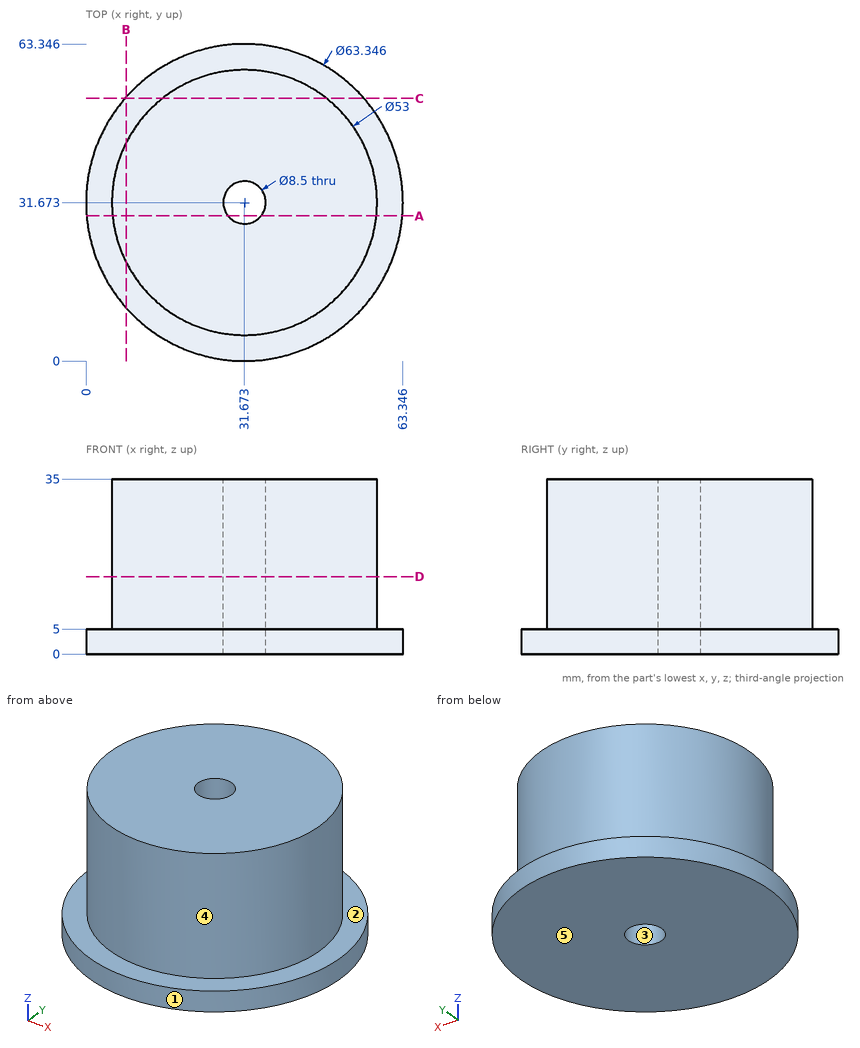
Study the drawing (mm; zero at the part's minimum x, y, z) and answer. A direction names the side the tool comes from. Give positions to 0.01 mm unless a question says otherwise; leave off trailing zeros. Loops run counter-clockwise (first coordinate to the right, second up) from the corner with the lowest first, then second, coordinate; pieces in that order, holes last. Notation, with made-up numbers: M 60,-28.5 L 109,-28.5 A16 ccw 109,-8.5 Z; hole C 81,13 d3. An arc over 180 degrees is marked long. One line per item, written item: value.
1. Section B-B on x = 8 is taken. Determine the outline of the cut face in (y, z).
Found:
outline: M 10.63,0 L 52.72,0 L 52.72,5 L 43.58,5 L 43.58,35 L 19.76,35 L 19.76,5 L 10.63,5 Z
2. For the marked faces 4 and 5, determine the directions among +Z, -Z, +X, -X, +Y, -Y from which every point of the face is accessible in a straight line to the end or side of a thin tool.
Found:
face 4: +Z
face 5: -Z, +X, -X, +Y, -Y
3. Section C-C on y = 52.5 is taken. Determine the outline of the cut face in (x, z).
Found:
outline: M 7.81,0 L 55.54,0 L 55.54,5 L 48.06,5 L 48.06,35 L 15.29,35 L 15.29,5 L 7.81,5 Z
4. Each of these flat-tipped pins is pushed along its axis until it touches: P1, Ø12, axis at x = 18, z = 13, coming from the -Y side; P2, Ø5, axis at y = 38, z = 16, coming from the -X side; P3, Ø6, axis at y = 51.5, z = 19, coming from the +X side (3 decimals). Where does it stop, or does it pass through?
Found:
P1: y = 6.31
P2: x = 5.45
P3: x = 52.145
5. For a pull along Y with two mould halves and no side action, classify the marked faces 1, 2 and 3 as pulls with the +Y half, pulls with the -Y half, needs draft (parallel to the pull), parting line crosses it, or undercut.
Found:
face 1: parting line crosses it
face 2: needs draft
face 3: undercut
6. Section D-D on z = 15.5 is taken. Determine the outline of the cut face in (x, y), plus the area to 3 significant figures.
Found:
outline: C 31.67,31.67 d53; hole C 31.67,31.67 d8.5
area: 2,150 mm^2
7. Find the intervals of material crossed by probe 1 along X at (y, z) = (31.5, 30); probe 2 along Z at (x, y) = (30, 60.5); probe 3 along X at (y, z) = (31, 24.5), in increasing order.
Found:
probe 1: 5.17 to 27.43, 35.92 to 58.17
probe 2: 0 to 5
probe 3: 5.18 to 27.48, 35.87 to 58.16
8. Section A-A on y = 29 is taken. Determine the outline of the cut face in (x, z), plus the area to 3 significant figures.
Found:
outline: M 0.11,0 L 28.37,0 L 28.37,35 L 5.31,35 L 5.31,5 L 0.11,5 Z; M 34.98,0 L 63.23,0 L 63.23,5 L 58.04,5 L 58.04,35 L 34.98,35 Z
area: 1,670 mm^2
